The model under review builds one solid part; all positions refer to its coordinate system, in mm. Give positions to 0.01 mm unless a question says otherwise; leave off trailing zeros. Loops run counter-clockwise (first coordinate to the right, second up) from the corner with the lowest first, then second, coordinate; pieces in that order, holes last. Notation, with made-up numbers: M 2.25,56 L 6.25,56 A21 ccw 6.25,95 Z; hole C 28,16 d9. An arc over 180 degrees is marked long. Put each result on its own line as item: value. Start each with the question number.
Autodesk Inventor part; units mm, degrees
ref_plane "YZ Plane" through (0, 0, 0) normal (1, 0, 0) x (0, 1, 0)
ref_plane "XZ Plane" through (0, 0, 0) normal (0, 1, 0) x (-1, 0, 0)
ref_plane "XY Plane" through (0, 0, 0) normal (0, 0, 1) x (1, 0, 0)
sketch "Sketch1" plane through (0, 0, 0) normal (0, 0, 1) x (1, 0, 0)
  line L0 (0, 0) -> (40, 0)
  line L1 (40, 0) -> (40, 20)
  line L2 (40, 20) -> (0, 20)
  line L3 (0, 20) -> (0, 0)
  line L4 (0, 10) -> (10, 10) construction
  line L5 (10, 10) -> (30, 10) construction
  circle A0 centre (10, 10) radius 2.55
  circle A1 centre (30, 10) radius 2.55
  line L6 (37.5, 0) -> (37.5, 20)
  line L7 (2.5, 0) -> (2.5, 20)
  dimension "d0" = 40
  dimension "d1" = 20
  dimension "d2" = 10
  dimension "d3" = 20
  dimension "d4" = 5.1
  dimension "d5" = 5.1
  dimension "d8" = 2.5
  dimension "d9" = 2.5
extrude "Extrusion1" add sketch "Sketch1" along normal blind 3 contours L7 L2 L6 L0
chamfer "Chamfer1" distance 3 angle 45 4 edges at (37.5, 0, 1.5) (37.5, 20, 1.5) (2.5, 20, 1.5) (2.5, 0, 1.5)
properties part number "Platinas de unión" material "Aluminum 6061"
Item 1: Consider section C-C, the plane z = 1.55. Write out the cut boundary in (x, y), plus the area to 3 significant figures.
Item 2: Clearance check with a flat-ended pin moving along its axis: pin 1 Ø3 at (x, y) = (10, 10) entering from -Z (1 decimal). State where the tip first meets the part, or that it passes through.
Item 3: To check wall thickness, follow L1, parallel to Y at x = 30, z = 0.6; L2, parallel to X at y = 9.25, z = 1.7; L3, parallel to X at y = 8.5, z = 0.55. State the ranges of each line that lie inside material, in increasing order. Write a range as [from, to].
Item 4: Draft analysis for pull direction Y (two halves, no side actions). For faces 1 (the cylindrical face through (27.976, 11.552, 1.479)), 2 (the flat face through (20, 10, 0)), 3 (the flat face through (36, 18.5, 1.5)), 4 (the cylindrical face through (11.18, 12.26, 1.48)), state which applies: +Y half, -Y half, draft (parallel to the pull), parting line (faces both ways), or undercut.
Item 5: Consider section D-D, the plane y = 18.75. Write out the cut boundary in (x, z), plus the area to 3 significant figures.
Item 6: Consider section B-B, the plane x = 30. Write out the cut boundary in (y, z).
Item 7: Consider section A-A, the plane y = 10. Write out the cut boundary in (x, z), plus the area to 3 significant figures.
Report:
1. outline: M 2.5,3 L 5.5,0 L 34.5,0 L 37.5,3 L 37.5,17 L 34.5,20 L 5.5,20 L 2.5,17 Z; hole C 10,10 d5.1; hole C 30,10 d5.1
1. area: 641 mm²
2. pin 1: through
3. L1: [0, 7.45], [12.55, 20]
3. L2: [2.5, 7.56], [12.44, 27.56], [32.44, 37.5]
3. L3: [2.5, 7.94], [12.06, 27.94], [32.06, 37.5]
4. face 1: undercut
4. face 2: draft
4. face 3: +Y half
4. face 4: undercut
5. outline: M 4.25,0 L 35.75,0 L 35.75,3 L 4.25,3 Z
5. area: 94.5 mm²
6. outline: M 0,0 L 7.45,0 L 7.45,3 L 0,3 Z; M 12.55,0 L 20,0 L 20,3 L 12.55,3 Z
7. outline: M 2.5,0 L 7.45,0 L 7.45,3 L 2.5,3 Z; M 12.55,0 L 27.45,0 L 27.45,3 L 12.55,3 Z; M 32.55,0 L 37.5,0 L 37.5,3 L 32.55,3 Z
7. area: 74.4 mm²
